Work out the finished part from the listing and answer in its coordinate system (mm). Face numbers are marked on the shaded views. A direction names the side the tool comes from. Round coordinates to 2 decimals unless told otherwise and drop trailing zeros. Loops run counter-clockwise (first coordinate to the right, second up) from the corner with the lowest first, then second, coordinate; pieces in that order, holes last. Notation, with made-up numbers: M 52.5,87 L 81.5,87 A22 cw 81.5,105 Z; hole C 43.5,32 d5. An arc over 180 degrees is marked long. One line per item, written item: value.
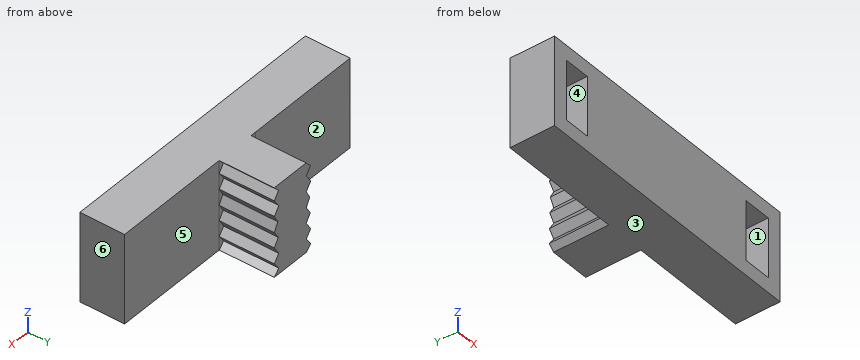
```python
from build123d import *

# Parameters (mm, degrees)
F1_DEPTH = 5
F2_DEPTH = 1
F4_DEPTH = 7.3914
F6_DEPTH = 7.39191


with BuildPart() as f1:
    # F0 (on Front) → F1 (new body)
    with BuildSketch(Plane.XZ):
        Polygon((-25.2447519526, 9.528346464), (12.7552480474, 9.528346464), (12.7552480474, 21.528346464), (7.0332471505, 21.528346464), (-19.9667528495, 21.528346464), (-25.2447519526, 21.528346464), align=None)
        Polygon((-19.7447519526, 11.528346464), (-23.2447519526, 11.528346464), (-23.2447519526, 19.528346464), (-19.7447519526, 19.528346464), (7.0332471505, 19.528346464), (10.7552480474, 19.528346464), (10.7552480474, 11.528346464), (7.0332471505, 11.528346464), align=None, mode=Mode.SUBTRACT)
        Polygon((-19.7447519526, 17.1880803001), (-19.7447519526, 11.528346464), (7.0332471505, 11.528346464), (7.0332471505, 13.5917593283), (7.0332471505, 19.528346464), (-19.7447519526, 19.528346464), align=None)
    extrude(amount=F1_DEPTH)

    # F0 (on Front) → F2 (join)
    with BuildSketch(Plane.XZ):
        Polygon((-25.2447519526, 9.528346464), (12.7552480474, 9.528346464), (12.7552480474, 21.528346464), (7.0332471505, 21.528346464), (-19.9667528495, 21.528346464), (-25.2447519526, 21.528346464), align=None)
        Polygon((-19.7447519526, 11.528346464), (-23.2447519526, 11.528346464), (-23.2447519526, 19.528346464), (-19.7447519526, 19.528346464), (7.0332471505, 19.528346464), (10.7552480474, 19.528346464), (10.7552480474, 11.528346464), (7.0332471505, 11.528346464), align=None, mode=Mode.SUBTRACT)
        Polygon((-19.7447519526, 17.1880803001), (-19.7447519526, 11.528346464), (7.0332471505, 11.528346464), (7.0332471505, 13.5917593283), (7.0332471505, 19.528346464), (-19.7447519526, 19.528346464), align=None)
        Polygon((7.0332471505, 13.5917593283), (7.0332471505, 11.528346464), (10.7552480474, 11.528346464), (10.7552480474, 19.528346464), (7.0332471505, 19.528346464), align=None)
        Polygon((-23.2447519526, 19.528346464), (-23.2447519526, 11.528346464), (-19.7447519526, 11.528346464), (-19.7447519526, 17.1880803001), (-19.7447519526, 19.528346464), align=None)
    extrude(amount=-F2_DEPTH)

    # F3 (on face) → F4 (join)
    with BuildSketch(Plane(origin=(0, 1, 0), x_dir=(-1, 0, 0), z_dir=(0, 1, 0))):
        Polygon((9.3062466048, 21.528346464), (3.1832573004, 21.528346464), (3.1832573004, 18.1184094399), (3.1832573004, 9.528346464), (9.3062466048, 9.528346464), (9.3062466048, 18.1184094399), align=None)
    extrude(amount=F4_DEPTH)

    # F5 (on face) → F6 (cut)
    with BuildSketch(Plane(origin=(0, 8.3914, 0), x_dir=(-1, 0, 0), z_dir=(0, 1, 0))):
        Polygon((9.3062466048, 21.528346464), (8.5453148931, 21.528346464), (9.2639319636, 20.7179207355), (8.5584444031, 19.7446867824), (9.3062466048, 18.6747785349), align=None)
        Polygon((9.3062466048, 12.255012989), (9.3062466048, 18.6171480624), (8.5584444031, 17.650116235), (9.1581455935, 16.5710970759), (8.5584444031, 15.4978624135), (9.242774643, 14.4342118874), (8.5584444031, 13.4398201481), align=None)
        Polygon((9.3062466048, 10.2662295103), (9.3062466048, 12.255012989), (8.5584444031, 11.3029358909), align=None)
        Polygon((9.3062466048, 9.528346464), (9.3062466048, 10.2662295103), (8.5881125659, 9.528346464), align=None)
        Polygon((3.9310595021, 10.2967135608), (3.1832573004, 11.3334199414), (3.1832573004, 9.528346464), align=None)
        Polygon((3.9310595021, 12.2854970396), (3.1832573004, 13.4703041986), (3.1832573004, 11.3334199414), align=None)
        Polygon((3.8675875403, 14.4646959379), (3.1832573004, 15.528346464), (3.1832573004, 13.4703041986), align=None)
        Polygon((3.7829584908, 16.6015811265), (3.1832573004, 17.6806002855), (3.1832573004, 15.528346464), align=None)
        Polygon((3.9522168227, 18.6749920249), (3.1832573004, 19.7751708329), (3.1832573004, 17.6806002855), align=None)
        Polygon((3.8887448609, 20.748404786), (3.1832573004, 21.528346464), (3.1832573004, 19.7751708329), align=None)
    extrude(amount=-F6_DEPTH, mode=Mode.SUBTRACT)


solid = f1.part
```
1) Each of these flat-tipped pins is pushed along its axis until it touches: pin 1 (3 mm diameter, centred on y = 3.5, z = 20, fed in from +X); pin 2 (4 mm diameter, centred on y = 4.5, z = 16.5, fed in from -X); pin 3 (3 mm diameter, centred on x = -15, z = 15.5, fed in from +Y); pin 4 (4 mm diameter, centred on x = -12.5, y = 3.5, fed in from +Z). Where does it stop, or does it pass through?
Check values:
pin 1: x = -3.18
pin 2: x = -9.22
pin 3: y = 1
pin 4: through
2) Find section B-B (x = 10). Give the vertices of the cut face in (y, z), then the cut area to 3 significant figures.
Check values:
outline: M -5,9.53 L 1,9.53 L 1,21.53 L -5,21.53 L -5,19.53 L 0,19.53 L 0,11.53 L -5,11.53 Z
area: 32.0 mm2
3) For the marked faces 1, 2 and 3, determine the directions among +Z, -Z, +X, -X, +Y, -Y from which every point of the face is accessible in a straight line to the end or side of a thin tool.
Check values:
face 1: -Y
face 2: +Z, -Z, -X, +Y
face 3: -Z, +X, -X, +Y, -Y
4) Find section A-A (y = -1). Give the vertices of the cut face in (x, z).
Check values:
outline: M -25.24,9.53 L 12.76,9.53 L 12.76,21.53 L -25.24,21.53 Z; hole M -23.24,11.53 L -19.74,11.53 L -19.74,19.53 L -23.24,19.53 Z; hole M 7.03,11.53 L 10.76,11.53 L 10.76,19.53 L 7.03,19.53 Z
5) Find the intervals of material crossed by probe 1 along X at (y, z) = (-2.5, 18.5); probe 2 along Z at (x, y) = (-20, -1); probe 3 along Y at (x, z) = (-22, 20.25), in increasing order. Write a range as from..to.
Check values:
probe 1: -25.24..-23.24, -19.74..7.03, 10.76..12.76
probe 2: 9.53..11.53, 19.53..21.53
probe 3: -5..1
6) The mould has two halves that part along X. Classify the marked faces 4, 5 and 6: +X half, -X half, draft (parallel to the pull), parting line (faces both ways), or undercut.
Check values:
face 4: undercut
face 5: draft
face 6: +X half
7) Find section D-D (x = -17). Give the vertices of the cut face in (y, z), then the cut area to 3 significant figures.
Check values:
outline: M -5,9.53 L 1,9.53 L 1,21.53 L -5,21.53 Z
area: 72.0 mm2
